Autodesk Inventor part; units mm, degrees
ref_plane "YZ Plane" through (0, 0, 0) normal (1, 0, 0) x (0, 1, 0)
ref_plane "XZ Plane" through (0, 0, 0) normal (0, 1, 0) x (-1, 0, 0)
ref_plane "XY Plane" through (0, 0, 0) normal (0, 0, 1) x (1, 0, 0)
sketch "Sketch3" plane through (0, 0, 0) normal (0, 0, 1) x (1, 0, 0)
  circle A0 centre (0, 0) radius 1.5
  dimension "Diameter" = 3
extrude "Extrusion1" add sketch "Sketch3" against normal blind 30
sketch "Sketch4" plane through (0, 0, 0) normal (0, 0, 1) x (1, 0, 0)
  circle A0 centre (0, 0) radius 1.5
  circle A1 centre (0, 0) radius 2.75
  dimension "Head_Diameter" = 5.5
extrude "Extrusion2" add sketch "Sketch4" along normal blind 3 contours A0 | A1
sketch "Sketch5" plane through (0, 0, 3) normal (0, 0, 1) x (1, 0, 0)
  circle A0 centre (0, 0) radius 2.75
  line L0 (1.4434, 0) -> (0.7217, -1.25)
  line L1 (0.7217, -1.25) -> (-0.7217, -1.25)
  line L2 (-0.7217, -1.25) -> (-1.4434, 0)
  line L3 (-1.4434, 0) -> (-0.7217, 1.25)
  line L4 (-0.7217, 1.25) -> (0.7217, 1.25)
  line L5 (0.7217, 1.25) -> (1.4434, 0)
  line L6 (0, 0) -> (1.4434, 0) construction
  dimension "Hex_Width" = 2.5
extrude "Extrusion3" cut sketch "Sketch5" against normal blind 1.5 contours L0 L1 L2 L3 L4 L5
thread "Thread1"
chamfer "Chamfer1" distance 0.3 angle 45 1 edges at (-2.75, 0, 3)
chamfer "Chamfer2" distance 0.15 angle 45 1 edges at (-1.5, 0, -30)
equation "\"d14\" = 0.5 * Chamfer"
properties part number "SCREW,SOCKET-HD,P,12_9,M03X0_5X30MM" material "Steel, MS"
The listing builds one solid part. Answer for the finished solid, in the listing's coordinates (mm). A direction names the side the tool comes from. Coordinates: 2 decimals unless noted, no trailing zeros. Loops run counter-clockwise (first coordinate to the right, second up) from the corner with the lowest first, then second, coordinate; pieces in that order, holes last. Notation, with made-up numbers: M -7,53 L 11,53 A16 cw 11,61 Z; hole C 79,-3.75 d11. An arc over 180 degrees is marked long. Answer as CSV lines item,"result". Start each with the question number.
(1) For faces 1 (the flat face through (-1.08, -0.63, 2.26)), 2 (the flat face through (1.2, -1.2, 0)), 3 (the cylindrical face through (-0.596, 2.685, 1.331)), determine the directions among +Z, -Z, +X, -X, +Y, -Y from which every point of the face is accessible in a straight line to the end or side of a thin tool.
(2) The part is cut by section A-A (x = 0). Give the vertices of the cut face in (y, z), and give its area (3 significant figures).
(3) The part is cut by section B-B (z = -1). Give the vertices of the cut face in (x, y).
(4) Given pin 1 (1 mm diameter, centred on y = -1, z = -18.5, fed in from -X); pin 2 (3 mm diameter, centred on x = 0, z = -5, fed in from -Y), each flat-ended and moving along its own axis, determine where each tip first touches the part or whether it passes through.
(5) Find the intervals of material crossed by L1, parallel to Z at x = -0.8, y = -2.1; L2, parallel to Z at x = -0.75, y = 0.9; L3, parallel to Y at x = -0.65, z = -24.5, in increasing order. Write a range as [from, to].
Determined:
1,face 1,"+Z"
1,face 2,"-Z"
1,face 3,"+Z, -Z"
2,outline,"M -2.75,0 L -1.5,0 L -1.5,-29.85 L -1.35,-30 L 1.35,-30 L 1.5,-29.85 L 1.5,0 L 2.75,0 L 2.75,2.7 L 2.45,3 L 1.25,3 L 1.25,1.5 L -1.25,1.5 L -1.25,3 L -2.45,3 L -2.75,2.7 Z"
2,area,"103 mm2"
3,outline,"C 0,0 d3"
4,pin 1,"x = -1.41"
4,pin 2,"y = -1.5"
5,L1,"[0, 3]"
5,L2,"[-30, 1.5]"
5,L3,"[-1.35, 1.35]"
